The model under review builds one solid part; all positions refer to its coordinate system, in mm. Face numbers are marked on the shaded views. A direction names the side the tool comes from. Round coordinates to 2 decimals unless told otherwise and drop trailing zeros. Order: outer loops, then holes, each group sorted by start corner. A loop starts at its lowest first (then second) coordinate and runs counter-clockwise, first axis right, second up. Notation, with made-up numbers: (63, -13.75) - (96, -13.75) arc R23 cw to (96, 21.25) - close; hole circle Ø3 at (85, 27). An arc over 180 degrees is marked (long way). One line per question, with ' | ' between items. Start each with the question number.
Item 1: Insertion check: pin 1 Ø2.5 at (y, z) = (39, 10) entering from +X; pin 2 Ø1.8 at (x, z) = (0.5, 14.5) entering from +Y; pin 3 Ø1 at (y, z) = (31, 16) entering from -X. Each pin has a flat end and moves straight along its axis. Give the tip position at first contact, or say it passes through.
Item 2: Draft analysis for pull direction X (two halves, no side actions). For the marked faces 4, 5 and 6, state which applies: +X half, -X half, draft (parallel to the pull), parting line (faces both ways), or undercut.
Item 3: Add section D-D on x = 23. State the section outline as (y, z) points.
Item 4: Add section A-A on z = 11. State the section outline as (x, y) points.
Item 5: For L1, parallel to X at y = 27, z = 18.25; L2, parallel to X at y = 39, z = 19; L3, parallel to X at y = 24.5, z = 11, list the stretches that pass through material, from the lowest coordinate up. Write a range as [from, to].
Item 6: Add section B-B on z = 7.25. State the section outline as (x, y) points, and give its area (3 significant figures).
Item 7: Add section C-C on y = 13. State the section outline as (x, z) points.
Item 8: Tool access review of the marked faces 1, 2 and 3: name each direction out of +Z, -Z, +X, -X, +Y, -Y from which nothing blocks a thin tool from reaching the whole face with its end or side.
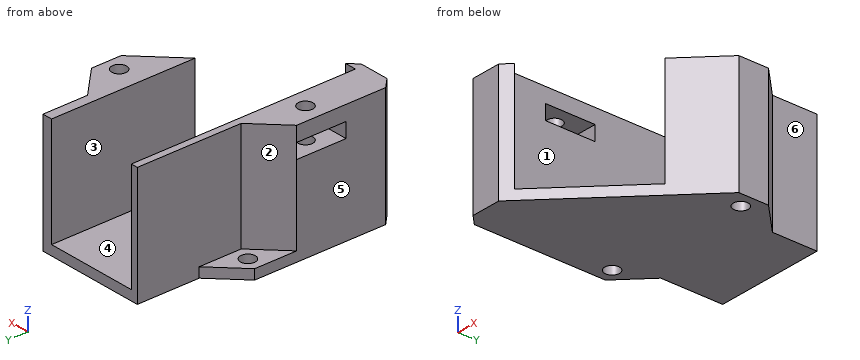
from build123d import *

# Parameters (mm, degrees)
SKETCH_R        = 1.5
PAD_DEPTH       = 2
PAD001_DEPTH    = 22
SKETCH002_R     = 1.5
POCKET_DEPTH    = 32
SKETCH003_R     = 1.5
POCKET001_DEPTH = 15
SKETCH004_W     = 10
SKETCH004_H     = 3
POCKET002_DEPTH = 8


with BuildPart() as part:
    # Sketch → Pad (new body)
    with BuildSketch(Plane.XY):
        Polygon((-6, -2), (0, -2), (20, 18), (26, 24), (26, 30), (20, 36), (20, 45), (-2, 45), (-2, 32.485281), (-8, 26.485281), (-8, 18), (-8, 0), align=None)
        with Locations((-5, 25.242641)):
            Circle(SKETCH_R, mode=Mode.SUBTRACT)
        with Locations((23, 27)):
            Circle(SKETCH_R, mode=Mode.SUBTRACT)
    extrude(amount=PAD_DEPTH)

    # Sketch001 (on Face16 of Pad) → Pad001 (join)
    with BuildSketch(Plane.XY.offset(2)):
        Polygon((-2, 32.485281), (-2, 45), (-0.6, 45), (-0.6, -0.3), (1.7, -0.3), (0, -2), (-6, -2), (-8, 0), (-8, 18), (-2, 24), align=None)
        Polygon((20, 45), (18, 45), (18, 16), (26, 24), (26, 30), (20, 36), align=None)
    extrude(amount=PAD001_DEPTH)

    # Sketch002 (on Face31 of Pad001) → Pocket (cut)
    with BuildSketch(Plane(origin=(0, 0, 2), x_dir=(1, 0, 0), z_dir=(0, 0, -1))):
        with Locations((23, -27)):
            Circle(SKETCH002_R)
    extrude(amount=-POCKET_DEPTH, mode=Mode.SUBTRACT)

    # Sketch003 (on Face19 of Pocket) → Pocket001 (cut)
    with BuildSketch(Plane.XY.offset(24)):
        with Locations((-4.3, 13)):
            Circle(SKETCH003_R)
    extrude(amount=-POCKET001_DEPTH, mode=Mode.SUBTRACT)

    # Sketch004 (on Face9 of Pocket001) → Pocket002 (cut)
    with BuildSketch(Plane(origin=(-8, 0, 0), x_dir=(0, -1, 0), z_dir=(-1, 0, 0))):
        with Locations((-13, 19.5)):
            Rectangle(SKETCH004_W, SKETCH004_H)
    extrude(amount=-POCKET002_DEPTH, mode=Mode.SUBTRACT)


solid = part.part
Determined:
1) pin 1: x = 20 | pin 2: y = -0.3 | pin 3: x = -2
2) face 4: undercut | face 5: -X half | face 6: +X half
3) outline: (21, 0) - (25.5, 0) - (25.5, 24) - (21, 24) - close; (28.5, 0) - (33, 0) - (33, 24) - (28.5, 24) - close
4) outline: (-8, 0) - (-6, -2) - (0, -2) - (1.7, -0.3) - (-0.6, -0.3) - (-0.6, 45) - (-2, 45) - (-2, 24) - (-8, 18) - close; (18, 16) - (26, 24) - (26, 30) - (20, 36) - (20, 45) - (18, 45) - close; hole circle Ø3 at (-4.3, 13); hole circle Ø3 at (23, 27)
5) L1: [-2, -0.6], [18, 21.5], [24.5, 26] | L2: [-2, -0.6], [18, 20] | L3: [-2, -0.6], [18, 26]
6) outline: (-8, 0) - (-6, -2) - (0, -2) - (1.7, -0.3) - (-0.6, -0.3) - (-0.6, 45) - (-2, 45) - (-2, 24) - (-8, 18) - close; (18, 16) - (26, 24) - (26, 30) - (20, 36) - (20, 45) - (18, 45) - close; hole circle Ø3 at (23, 27) | area: 325 mm2
7) outline: (-8, 0) - (15, 0) - (15, 2) - (-0.6, 2) - (-0.6, 18) - (-2.8, 18) - (-2.8, 9) - (-5.8, 9) - (-5.8, 18) - (-8, 18) - close; (-8, 21) - (-5.8, 21) - (-5.8, 24) - (-8, 24) - close; (-2.8, 21) - (-0.6, 21) - (-0.6, 24) - (-2.8, 24) - close
8) face 1: +Z, +Y | face 2: +Z, -X, +Y | face 3: +Z, +Y, -Y
